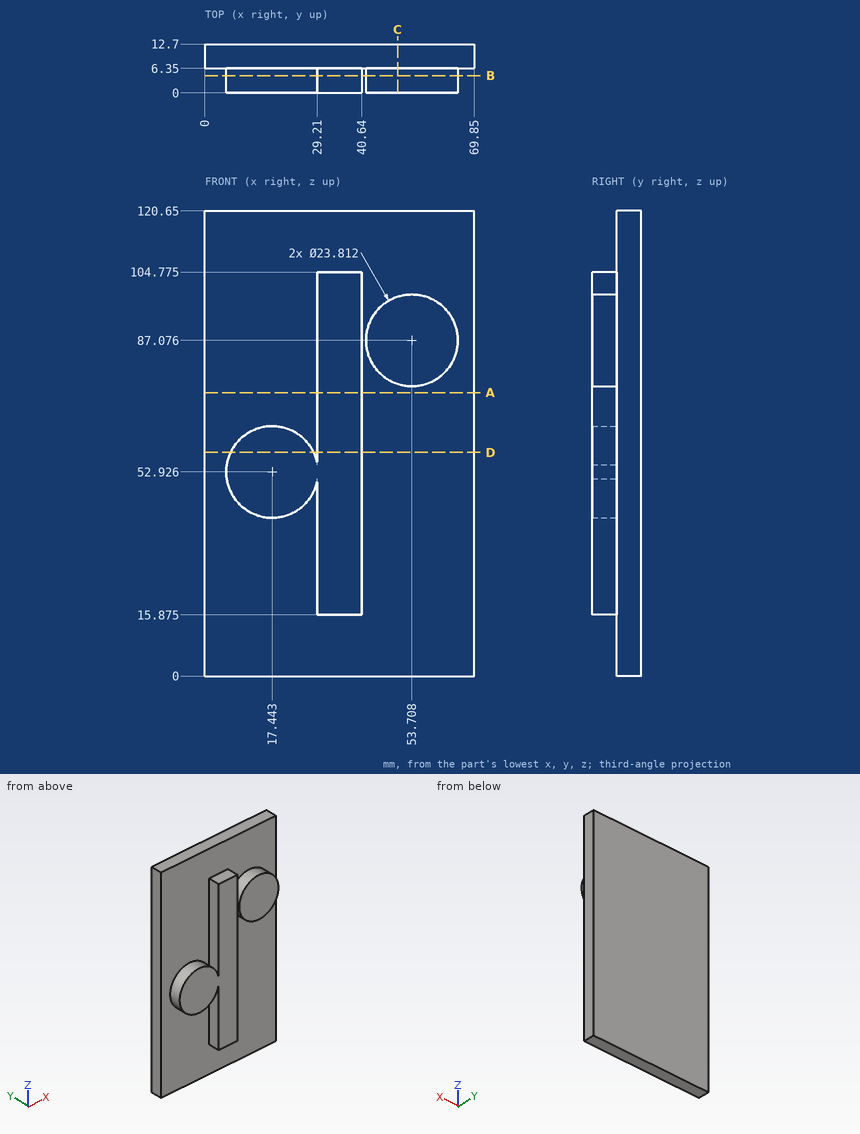
Verification items for this drawing (mm, ordinates from the low corner). Coordinates: 2 decimals unless noted, no trailing zeros. Write each loop counter-clockwise with the first axis right and the second up, starting at its lowest first coordinate (ties: lowest second). Pieces come first, ordered by that corner, then holes. Notation, with made-up numbers: M 69,1.5 L 124,1.5 A23 ccw 124,30.5 Z; hole C -20,83.25 d3. An arc over 180 degrees is marked long. Answer as a JSON object with one key per item and string values.
1. Go/stop test with flat-tipped pins: pin 1 Ø1.9 at (y, z) = (3.5, 80) entering from +X; pin 2 Ø3 at (x, z) = (61.5, 60.5) entering from -Y; pin 3 Ø3 at (x, y) = (34, 4.5) entering from -Z (1 decimal). Record where each tip stops, or that it passes through.
Answers below:
{"pin 1": "stops at x = 63.92", "pin 2": "stops at y = 6.35", "pin 3": "stops at z = 15.9"}
2. Section check B-B, the plane y = 4.5. Enter the section's corners in (x, z) (1 decimal), plus the area to 3 significant figures.
Answers below:
{"outline": "M 29.2,15.9 L 40.6,15.9 L 40.6,104.8 L 29.2,104.8 L 29.2,54.7 A11.9 ccw long 29.2,51.1 Z; C 53.7,87.1 d23.8", "area": "1,910 mm²"}
3. Section check C-C, the plane x = 50. Enter the section's corners in (y, z).
Answers below:
{"outline": "M 0,75.76 L 6.35,75.76 L 6.35,0 L 12.7,0 L 12.7,120.65 L 6.35,120.65 L 6.35,98.39 L 0,98.39 Z"}
4. Scan lines: L1, parallel to Y at x = 6, z = 16; L2, parallel to X at y = 6.25, z = 61 (1 decimal); L3, parallel to X at y = 2, z = 34. Record each from-to range of solid material in increasing order.
Answers below:
{"L1": "y = 6.35 to 12.7", "L2": "x = 8.7 to 26.2, 29.2 to 40.6", "L3": "x = 29.21 to 40.64"}
5. Section check A-A, the plane z = 73.5. Enter the section's corners in (x, y), plus the area to 3 significant figures.
Answers below:
{"outline": "M 0,6.35 L 29.21,6.35 L 29.21,0 L 40.64,0 L 40.64,6.35 L 69.85,6.35 L 69.85,12.7 L 0,12.7 Z", "area": "516 mm²"}
6. Section check D-D, the plane z = 58. Enter the section's corners in (x, y).
Answers below:
{"outline": "M 0,6.35 L 6.67,6.35 L 6.67,0 L 28.21,0 L 28.21,6.35 L 29.21,6.35 L 29.21,0 L 40.64,0 L 40.64,6.35 L 69.85,6.35 L 69.85,12.7 L 0,12.7 Z"}
